from build123d import *

# Parameters (mm, degrees)
F1_DEPTH = 101.6
F2_W     = 50.8
F2_H     = 25.4
F3_DEPTH = 25.4


with BuildPart() as f1:
    # F0 (on Right) → F1 (new body)
    with BuildSketch(Plane.YZ):
        Polygon((50.8000037106, 12.7), (50.8000037106, 50.8), (0, 0), (38.1, 0), (38.1, 12.7030098811), align=None)
    extrude(amount=F1_DEPTH)

    # F2 (on Top) → F3 (join)
    with BuildSketch(Plane.XY):
        with Locations((25.4, 12.7)):
            Rectangle(F2_W, F2_H)
    extrude(amount=F3_DEPTH)


solid = f1.part
Input: part model. Units: mm. Frame: model coordinates. A direction names the side the tool comes from. Give positions to 0.01 mm unless a question says otherwise; leave off trailing zeros. Order: outer loops, then holes, each group sorted by start corner. A loop starts at its lowest first (then second) coordinate and runs counter-clockwise, first axis right, second up. Notation, with made-up numbers: (-24.75, 81) - (16.25, 81) arc R16 ccw to (16.25, 112) - close; hole circle Ø10 at (81.25, 1.25). An arc over 180 degrees is marked (long way). Write each question's results on one line, items separated by ' | '.
Item 1: Access query for faces 1 (the flat face through (50, 38.1, 6)), 2 (the flat face through (50, 50.8, 31)), 3 (the flat face through (50.8, 10, 15)), 4 (the flat face through (25, 13, 25.4)). Directions: +Z, -Z, +X, -X, +Y, -Y. A direction counts if a zero-diameter tool reaches every point of the face in a straight line with its end or side. Return the directions, or none.
A:
face 1: -Z, +X, -X, +Y | face 2: +Z, -Z, +X, -X, +Y | face 3: +Z, +X, -Y | face 4: +Z, +X, -X, -Y
Item 2: Section B-B (y = 20). Return loops of the section in (x, z).
A:
outline: (0, 0) - (101.6, 0) - (101.6, 20) - (50.8, 20) - (50.8, 25.4) - (0, 25.4) - close
Item 3: Section D-D (x = 61). Return loops of the section in (y, z), and give its area (3 significant figures).
A:
outline: (0, 0) - (38.1, 0) - (38.1, 12.7) - (50.8, 12.7) - (50.8, 50.8) - close | area: 1,130 mm^2
Item 4: Material intervals for line 1 along Z through (x, y) = (15, 19.5); line 2 along Z through (x, y) = (55, 27.5); line 3 along Y through (x, z) = (91, 30.5), sorted ascending.
A:
line 1: z = 0 to 25.4 | line 2: z = 0 to 27.5 | line 3: y = 30.5 to 50.8
Item 5: Contact query for flat-ended pins moving along their axis: pin 1 Ø1 at (y, z) = (27.5, 19) entering from -X; pin 2 Ø12 at (x, z) = (72.5, 33) entering from -Y; pin 3 Ø4 at (x, y) = (48.5, 27.5) entering from +Z; pin 4 Ø1.5 at (x, y) = (87, 14.5) entering from +Z. Output: stop coordinate, or through.
A:
pin 1: stops at x = 0 | pin 2: stops at y = 27 | pin 3: stops at z = 29.5 | pin 4: stops at z = 15.25
Item 6: Section C-C (z = 11). Return loops of the section in (x, y), and give its area (3 significant figures).
A:
outline: (0, 0) - (50.8, 0) - (50.8, 11) - (101.6, 11) - (101.6, 38.1) - (0, 38.1) - close | area: 3,310 mm^2
